Work out the finished part from the listing and answer in its coordinate system (mm). Face numbers are marked on the shaded views. A direction names the side the tool comes from. Coordinates: 2 decimals unless noted, no trailing zeros. Write each loop counter-clockwise with the first axis right and the second up, starting at its lowest first coordinate (ties: lowest second). Pieces come first, ordered by that corner, then holes. Notation, with made-up numbers: (22.5, -15.5) - (69.5, -15.5) arc R16 cw to (69.5, 15.5) - close; hole circle Ø8 at (64, -8). An arc over 180 degrees is marked (long way). Use one line per item in the form item = value. Start each with the question number.
Item 1: A cutting plane is placed at B-B (z = 7.5). Write down the section's boundary in (x, y), then the cut area to 3 significant figures.
Item 2: A cutting plane is placed at C-C (z = 1.5). Write down the section's boundary in (x, y), then the cut area to 3 significant figures.
Item 3: Given pin 1 (3 mm diameter, centred on x = -19, z = 5, fed in from -Y); pin 2 (1.5 mm diameter, centred on x = 1.5, z = 12.5, fed in from +Y), each flat-ended and moving along its own axis, determine where each tip first touches the part or whether it passes through.
Item 4: Determine the mould class of the marked faces 1, 2 and 3 for opening direction Z: released by +Z, released by -Z, zero draft, split by the parting line, or undercut.
Item 5: A cutting plane is placed at A-A (y = 8). Write down the section's boundary in (x, z), then the cut area to 3 significant figures.
Item 6: Consider probe 1 along X at (y, z) = (1.25, 6.75); probe 2 along X at (y, z) = (-2.25, 7.5); probe 3 along Y at (x, z) = (-19, 4). Determine where each line is inside the solid, lowest interval first.
Item 7: For the marked faces 4 and 5, determine the directions among +Z, -Z, +X, -X, +Y, -Y from which every point of the face is accessible in a straight line to the end or side of a thin tool.
Item 8: A cutting plane is placed at D-D (y = 1.5). Write down the section's boundary in (x, z).
from build123d import *

# Parameters (mm, degrees)
F1_DEPTH       = 15
F2_DEPTH       = 5
F3_DEPTH       = 5
F5_D           = 5
F5_CBORE_D     = 10
F5_CBORE_DEPTH = 8
F6_T1_DEPTH    = 66.4336597593
F7_R           = 2
F8_W           = 54.7069119513
F8_H           = 16.1263942719
F9_DEPTH       = 1


# Not quite as in the source:
# - a fillet or chamfer that OpenCascade refuses, or shapes differently, is made with other operations: its cross-section is extruded or revolved along the edge and cut away or added


with BuildPart() as f1:
    # F0 (on Top) → F1 (new body)
    with BuildSketch(Plane.XY):
        with BuildLine():
            Line((-21, -10), (21, -10))
            Line((21, -10), (21, 10))
            Line((21, 10), (11.1552678139, 10))
            ThreePointArc((11.1552678139, 10), (0, -0.2), (-11.1552678139, 10))
            Line((-11.1552678139, 10), (-21, 10))
            Line((-21, 10), (-21, -10))
        make_face()
    extrude(amount=F1_DEPTH)

    # F2 (add): a face of the model
    f2_faces = [f1.faces().sort_by_distance(p)[0] for p in [
        (21, 0, 7.5),
    ]]
    extrude(f2_faces, amount=F2_DEPTH)

    # F3 (add): a face of the model
    f3_faces = [f1.faces().sort_by_distance(p)[0] for p in [
        (-21, 0, 7.5),
    ]]
    extrude(f3_faces, amount=F3_DEPTH)

    # F5 (through all)
    with Locations(Plane.XZ.offset(10)):
        with Locations((18.577633907, 7.5), (-18.577633907, 7.5)):
            CounterBoreHole(F5_D / 2, F5_CBORE_D / 2, F5_CBORE_DEPTH)

    # F6: chamfer of 10 on 2 edges, made by hand

    # F6_s2 → F6_t1 (cut)
    with BuildSketch(Plane.XY.offset(-25.7168298797)):
        Polygon((16, -10), (26, 0), (26, -10), align=None)
        Polygon((-26, 0), (-16, -10), (-26, -10), align=None)
    extrude(amount=F6_T1_DEPTH, mode=Mode.SUBTRACT)

    # F7
    f7_edges = [f1.edges().sort_by_distance(p)[0] for p in [
        (0, -10, 15),
        (21, -5, 15),
        (-26, 5, 15),
        (26, 5, 15),
        (-21, -5, 15),
        (21, -5, 0),
        (0, -10, 0),
        (-21, -5, 0),
        (26, 5, 0),
        (-26, 5, 0),
        (16, -10, 13.392184),
        (16, -10, 1.607816),
        (-16, -10, 1.607816),
        (-16, -10, 13.392184),
        (26, 0, 7.5),
        (-26, 0, 7.5),
    ]]
    fillet(f7_edges, radius=F7_R)

    # F8 (on face) → F9 (cut)
    with BuildSketch(Plane(origin=(0, 10, 0), x_dir=(-1, 0, 0), z_dir=(0, 1, 0))):
        with Locations((-1.3534559757, 8.0631971359)):
            Rectangle(F8_W, F8_H)
    extrude(amount=-F9_DEPTH, mode=Mode.SUBTRACT)


solid = f1.part
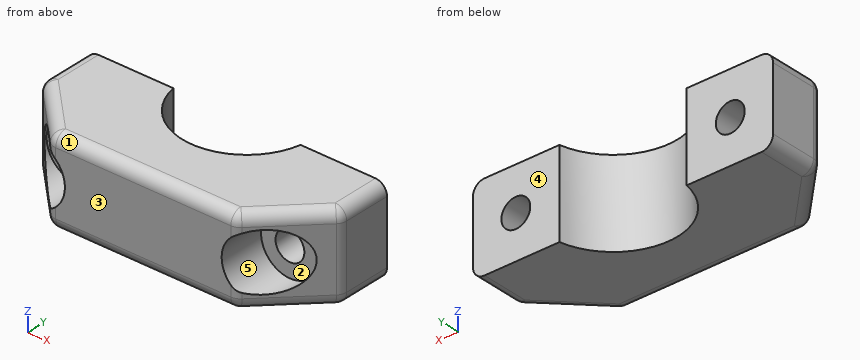
Answer:
q1.outline = (-26, 0.83) arc R2 ccw to (-25.41, -0.59) - (-23.58, -2.42) - (-23.58, -2) - (-21.08, -2) - (-21.08, 9) - (-26, 9) - close; (-16.08, -2) - (-13.58, -2) - (-13.58, -10) - (13.58, -10) - (13.58, -2) - (16.08, -2) - (16.08, 9) - (11.02, 9) arc R11.2 cw to (-11.02, 9) - (-16.08, 9) - close; (21.08, -2) - (23.58, -2) - (23.58, -2.42) - (25.41, -0.59) arc R2 ccw to (26, 0.83) - (26, 9) - (21.08, 9) - close
q1.area = 523 mm²
q2.outline = (-25.94, 0.83) arc R1.94 ccw to (-25.37, -0.54) - (-16.54, -9.37) arc R1.94 ccw to (-15.17, -9.94) - (15.17, -9.94) arc R1.94 ccw to (16.54, -9.37) - (25.37, -0.54) arc R1.94 ccw to (25.94, 0.83) - (25.94, 9) - (11.02, 9) arc R11.2 cw to (-11.02, 9) - (-25.94, 9) - close
q2.area = 730 mm²
q3.pin_1 = -2
q3.pin_2 = 0.03
q4.face_1 = released by +Z
q4.face_2 = undercut
q4.face_3 = zero draft
q5.outline = (-26, 2) arc R2 ccw to (-24, 0) - (-10.79, 0) - (-10.79, 15) - (-24, 15) arc R2 ccw to (-26, 13) - close; (10.79, 0) - (24, 0) arc R2 ccw to (26, 2) - (26, 13) arc R2 ccw to (24, 15) - (10.79, 15) - close; hole circle Ø5 at (-18.58, 7.5); hole circle Ø5 at (18.58, 7.5)
q5.area = 414 mm²
q6.probe_1 = -26 to -20.96, -16.19 to -5.51, 5.51 to 16.19, 20.96 to 26
q6.probe_2 = -23.75 to -23.58, -13.58 to 13.58, 23.58 to 23.75
q6.probe_3 = -2 to 9
q7.face_4 = +Z, -Z, +X, -X, +Y
q7.face_5 = -Y
q8.outline = (-26, 2) arc R2 ccw to (-24, 0) - (-5.93, 0) - (-5.93, 15) - (-24, 15) arc R2 ccw to (-26, 13) - close; (5.93, 0) - (24, 0) arc R2 ccw to (26, 2) - (26, 13) arc R2 ccw to (24, 15) - (5.93, 15) - close; hole circle Ø5 at (-18.58, 7.5); hole circle Ø5 at (18.58, 7.5)
